from build123d import *

# Parameters (mm, degrees)
F0_W          = 38.1
F0_H          = 609.6
F0_R          = 6.35
F1_DEPTH      = 3.175
F2_DEPTH      = 76.2
F2_DEPTH_BACK = 3.175
F3_DEPTH      = 25.4


with BuildPart() as f1:
    # F0 (on Front) → F1 (new body)
    with BuildSketch(Plane.XZ):
        with Locations((19.05, 304.8)):
            Rectangle(F0_W, F0_H)
        with Locations((19.05, 25.4)):
            Circle(F0_R, mode=Mode.SUBTRACT)
        with Locations((19.05, 584.2)):
            Circle(F0_R, mode=Mode.SUBTRACT)
    extrude(amount=F1_DEPTH)

    # F0 (on Front) → F2 (join, two sides)
    with BuildSketch(Plane.XZ) as f2_sk:
        with Locations((19.05, 25.4)):
            Circle(F0_R)
    extrude(amount=F2_DEPTH)
    extrude(f2_sk.sketch, amount=-F2_DEPTH_BACK)

    # F0 (on Front) → F3 (join)
    with BuildSketch(Plane.XZ):
        with Locations((19.05, 584.2)):
            Circle(F0_R)
    extrude(amount=F3_DEPTH)


solid = f1.part
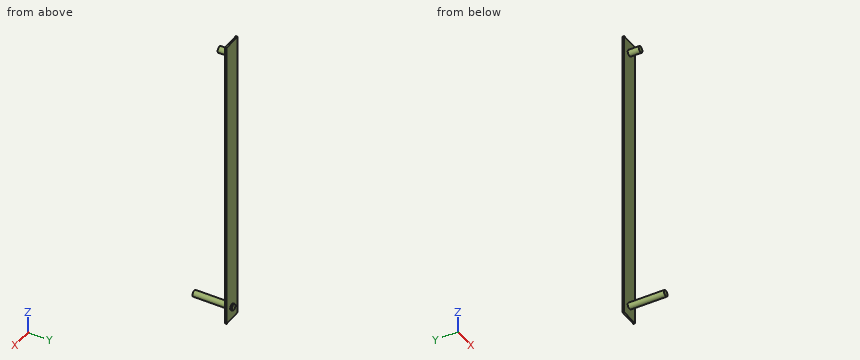
The listing builds one solid part. Answer for the finished solid, in the listing's coordinates (mm). Coordinates: 2 decimals unless noted, no trailing zeros. Order: outer loops, then holes, each group sorted by start corner. A loop starts at its lowest first (then second) coordinate and runs counter-clockwise, first axis right, second up.
Q1. Given P1, Ø12, axis at x = 28, y = -21, coming from the +Z side; P2, Ø4, axis at x = 32.5, z = 308.5, coming from the +Y side; P3, Ø1.5, axis at x = 27, y = -10, coming from the +Z side; P4, Ø1.5, axis at x = 18, z = 518, coming from the -Y side (3 decimals), each flat-ended and moving along its own axis, determine where each tip first touches the part or whether it passes through.
Q2. A cutting plane is placed at D-D, the plane y = -54. Write down the section's boundary in (x, z), and give its area (3 significant figures).
Q3. A cutting plane is placed at B-B, the plane x = 19.05. Write down the section's boundary in (y, z) (3 decimals), and give its area (3 significant figures).
Q4. A cutting plane is placed at C-C, the plane z = 584.2. Write down the section's boundary in (x, y) (3 decimals).
Q5. Consider line 1 (Z direction, x = 20, y = -15); line 2 (X direction, y = -16, z = 583); line 3 (Y direction, x = 13, z = 102) (3 decimals). Determine where each line is inside the solid, lowest interval first.
Q6. A cutting plane is placed at A-A, the plane y = -17. Write down the section's boundary in (x, z), and give its area (3 significant figures).
Answers follow:
1. P1: stops at z = 589.82
1. P2: stops at y = 0
1. P3: passes through
1. P4: stops at y = -3.175
2. outline: circle Ø12.7 at (19.05, 25.4)
2. area: 127 mm2
3. outline: (-76.2, 19.05) - (-3.175, 19.05) - (-3.175, 0) - (0, 0) - (0, 19.05) - (3.175, 19.05) - (3.175, 31.75) - (0, 31.75) - (0, 609.6) - (-3.175, 609.6) - (-3.175, 590.55) - (-25.4, 590.55) - (-25.4, 577.85) - (-3.175, 577.85) - (-3.175, 31.75) - (-76.2, 31.75) - close
3. area: 3,190 mm2
4. outline: (0, -3.175) - (12.7, -3.175) - (12.7, -25.4) - (25.4, -25.4) - (25.4, -3.175) - (38.1, -3.175) - (38.1, 0) - (0, 0) - close
5. line 1: z = 19.12 to 31.68, 577.92 to 590.48
5. line 2: x = 12.81 to 25.29
5. line 3: y = -3.175 to 0
6. outline: circle Ø12.7 at (19.05, 25.4); circle Ø12.7 at (19.05, 584.2)
6. area: 253 mm2
